Autodesk Inventor part; units mm, degrees
ref_plane "YZ Plane" through (0, 0, 0) normal (1, 0, 0) x (0, 1, 0)
ref_plane "XZ Plane" through (0, 0, 0) normal (0, 1, 0) x (-1, 0, 0)
ref_plane "XY Plane" through (0, 0, 0) normal (0, 0, 1) x (1, 0, 0)
sketch "Sketch1" plane through (0, 0, 0) normal (0, 1, 0) x (-1, 0, 0)
  line L0 (0.3746, 1.6788) -> (0.3747, -4.4196)
  line L1 (3.5497, -7.5946) -> (5.0483, -7.5946)
  arc A0 (7.6772, -6.364) -> (5.0483, -6.4323) centre (6.3183, -4.6863) ccw
  line L2 (7.6772, -7.5946) -> (20.7963, -7.5946)
  arc A1 (23.4251, -6.4323) -> (20.7962, -6.364) centre (22.1552, -4.6863) ccw
  line L3 (23.4252, -7.5946) -> (24.9238, -7.5946)
  line L4 (20.7963, 66.2432) -> (7.6772, 66.2432)
  arc A2 (5.0483, 65.0809) -> (7.6772, 65.0126) centre (6.3183, 63.3349) ccw
  line L5 (5.0483, 66.2432) -> (3.5496, 66.2432)
  line L6 (24.9237, 66.2432) -> (23.4252, 66.2432)
  arc A3 (20.7962, 65.0126) -> (23.4251, 65.0809) centre (22.1552, 63.3349) ccw
  circle A4 centre (14.2367, 45.0719) radius 6.9278
  arc A5 (1.9876, 15.9067) -> (5.1626, 12.7318) centre (5.1626, 15.9067) ccw
  line L7 (5.1626, 12.7318) -> (23.3109, 12.7318)
  arc A6 (23.3109, 12.7318) -> (26.4859, 15.9068) centre (23.3109, 15.9068) ccw
  line L8 (26.4859, 15.9068) -> (26.4859, 45.1707)
  arc A7 (26.4859, 45.1707) -> (1.9876, 45.1707) centre (14.2367, 45.0719) ccw
  line L9 (1.9876, 45.1707) -> (1.9876, 15.9067)
  arc A8 (27.813, 45.1759) -> (0.6604, 45.1759) centre (14.2367, 45.0719) ccw
  circle A9 centre (14.2367, 45.0719) radius 6.9278
  line L10 (0.3746, 66.2432) -> (13.2207, 66.2432)
  line L11 (13.2207, 66.2432) -> (13.2207, 60.019)
  line L12 (13.2207, 60.019) -> (0.3746, 60.019)
  line L13 (0.3746, 60.019) -> (0.3746, 66.2432)
  line L14 (0.3746, 60.019) -> (13.2207, 60.019)
  line L15 (13.2207, 60.019) -> (13.2207, 59.1663)
  line L16 (13.2207, 59.1663) -> (0.3746, 59.1663)
  line L17 (0.3746, 59.1663) -> (0.3746, 60.019)
  line L18 (14.2367, 45.0719) -> (14.2367, 66.2432)
  line L19 (28.0988, 66.2432) -> (15.2527, 66.2432)
  line L20 (15.2527, 66.2432) -> (15.2527, 60.019)
  line L21 (28.0988, 60.019) -> (28.0988, 66.2432)
  line L22 (28.0988, 60.019) -> (15.2527, 60.019)
  line L23 (15.2527, 60.019) -> (15.2527, 59.1663)
  line L24 (15.2527, 59.1663) -> (28.0988, 59.1663)
  line L25 (28.0988, 59.1663) -> (28.0988, 60.019)
  circle A10 centre (6.3183, 63.3349) radius 2.159
  circle A11 centre (22.1552, 63.3349) radius 2.159
  line L26 (0.3746, 66.2432) -> (0.3746, -7.5946)
  line L27 (0.3746, 29.3243) -> (28.0988, 29.3243)
  line L28 (20.7963, -7.5946) -> (7.6772, -7.5946)
  arc A12 (7.6772, -6.364) -> (5.0483, -6.4323) centre (6.3182, -4.6863) ccw
  line L29 (5.0483, -7.5946) -> (3.5497, -7.5946)
  line L30 (24.9238, -7.5946) -> (23.4252, -7.5946)
  arc A13 (23.4251, -6.4323) -> (20.7962, -6.364) centre (22.1551, -4.6863) ccw
  line L31 (0.3746, -7.5946) -> (13.2207, -7.5946)
  line L32 (13.2207, -7.5946) -> (13.2207, -1.3704)
  line L33 (13.2207, -1.3704) -> (0.3746, -1.3704)
  line L34 (0.3746, -1.3704) -> (0.3746, -7.5946)
  line L35 (0.3746, -1.3704) -> (13.2207, -1.3704)
  line L36 (13.2207, -1.3704) -> (13.2207, -0.5177)
  line L37 (13.2207, -0.5177) -> (0.3746, -0.5177)
  line L38 (0.3746, -0.5177) -> (0.3746, -1.3704)
  line L39 (28.0988, -1.3704) -> (28.0988, -7.5946)
  line L40 (28.0988, -7.5946) -> (15.2527, -7.5946)
  line L41 (15.2527, -7.5946) -> (15.2527, -1.3704)
  line L42 (28.0988, -1.3704) -> (15.2527, -1.3704)
  line L43 (15.2527, -0.5177) -> (28.0988, -0.5177)
  line L44 (15.2527, -1.3704) -> (15.2527, -0.5177)
  line L45 (28.0988, -0.5177) -> (28.0988, -1.3704)
  circle A14 centre (6.3182, -4.6863) radius 2.159
  circle A15 centre (22.1551, -4.6863) radius 2.159
  line L46 (28.0988, -7.5946) -> (15.2527, -7.5946)
  line L47 (15.2527, -7.5946) -> (15.2527, -1.3704)
  line L48 (15.2527, -1.3704) -> (28.0988, -1.3704)
  line L49 (28.0988, -1.3704) -> (28.0988, -7.5946)
  line L50 (13.2207, -7.5946) -> (0.3746, -7.5946)
  line L51 (0.3746, -7.5946) -> (0.3746, -1.3704)
  line L52 (0.3746, -1.3704) -> (13.2207, -1.3704)
  line L53 (13.2207, -1.3704) -> (13.2207, -7.5946)
  line L54 (28.0988, 66.2432) -> (15.2527, 66.2432)
  line L55 (15.2527, 66.2432) -> (15.2527, 60.019)
  line L56 (15.2527, 60.019) -> (28.0988, 60.019)
  line L57 (28.0988, 60.019) -> (28.0988, 66.2432)
  point P0 (0, 0)
  point P1 (0, 20.6785)
  point P2 (14.2367, -7.5946)
extrude "Extrusion1" add sketch "Sketch1" along normal blind 1 contours L41 L42 L39 L40 L3 L2 | L4 L19 L6 L21 L22 L20 | L33 L32 L2 L31 L1 L26 L0 | L13 L10 L5 L4 L11 L12
sketch "Sketch2" plane through (0, 0, 0) normal (0, -1, 0) x (1, 0, 0)
  circle A0 centre (-22.1552, 63.3349) radius 2.159
  line L0 (-28.0988, 66.2432) -> (-15.2527, 66.2432)
  line L1 (-28.0988, 60.019) -> (-28.0988, 66.2432)
  line L2 (-15.2527, 60.019) -> (-28.0988, 60.019)
  line L3 (-15.2527, 66.2432) -> (-15.2527, 60.019)
  circle A1 centre (-6.3183, 63.3349) radius 2.159
  line L4 (-0.3746, 66.2432) -> (-0.3746, 60.019)
  line L5 (-13.2207, 66.2432) -> (-0.3746, 66.2432)
  line L6 (-13.2207, 60.019) -> (-13.2207, 66.2432)
  line L7 (-0.3746, 60.019) -> (-13.2207, 60.019)
  circle A2 centre (-22.1551, -4.6863) radius 2.159
  line L8 (-15.2527, -1.3704) -> (-15.2527, -7.5946)
  line L9 (-28.0988, -1.3704) -> (-15.2527, -1.3704)
  line L10 (-28.0988, -7.5946) -> (-28.0988, -1.3704)
  line L11 (-15.2527, -7.5946) -> (-28.0988, -7.5946)
  line L12 (-28.0988, 60.019) -> (-0.3746, 60.019)
  line L13 (-0.3746, 60.019) -> (-0.3746, 59.13)
  line L14 (-0.3746, 59.13) -> (-28.0988, 59.13)
  line L15 (-28.0988, 59.13) -> (-28.0988, 60.019)
  line L16 (-28.0988, -1.3704) -> (-0.3746, -1.3704)
  line L17 (-0.3746, -1.3704) -> (-0.3746, -0.4814)
  line L18 (-0.3746, -0.4814) -> (-28.0988, -0.4814)
  line L19 (-28.0988, -0.4814) -> (-28.0988, -1.3704)
  point P0 (0, 0)
  dimension "d2" = 0.889
  dimension "d3" = 0.889
extrude "Extrusion2" add sketch "Sketch2" against normal blind 8.8392 contours L2 L12 L7 L13 L14 L15 | L9 L19 L18 L17 L16
sketch "Sketch3" plane through (0, 8.8392, 0) normal (0, 1, 0) x (1, 0, 0)
  line L0 (-0.3746, 1.3704) -> (-28.0988, 1.3704)
  line L1 (-28.0988, 1.3704) -> (-28.0988, -60.019)
  line L2 (-28.0988, -60.019) -> (-0.3746, -60.019)
  line L3 (-0.3746, -60.019) -> (-0.3746, 1.3704)
  point P0 (0, 0)
extrude "Extrusion3" add sketch "Sketch3" along normal blind 1
fillet "Fillet1" radius 2.032 8 edges at (-28.0988, 0.5, 66.2432) (-15.2527, 0.5, 66.2432) (-13.2207, 0.5, 66.2432) (-0.3746, 0.5, 66.2432) (-0.3746, 0.5, -7.5946) (-13.2207, 0.5, -7.5946) (-15.2527, 0.5, -7.5946) (-28.0988, 0.5, -7.5946)
fillet "Fillet2" radius 1.016 4 edges at (-13.2207, 0.5, -1.3704) (-15.2527, 0.5, -1.3704) (-15.2527, 0.5, 60.019) (-13.2207, 0.5, 60.019)
extrude "Extrusion4" cut sketch "Sketch1" along normal blind 127 contours A4
sketch "Sketch4" plane through (0, 9.8392, 0) normal (0, 1, 0) x (1, 0, 0)
  circle A0 centre (-14.2367, -45.0719) radius 6.9278
  line L0 (-28.0988, 1.3704) -> (-28.0988, -60.019)
  circle A1 centre (-14.2367, -45.0719) radius 4.0005
  circle A2 centre (-14.2367, -13.0679) radius 4.0005
  line L1 (-14.2367, -13.0679) -> (-14.2367, -5.0669)
  circle A3 centre (-14.2367, -5.0669) radius 1.8542
  circle A4 centre (-22.2377, -13.0679) radius 1.8542
  circle A5 centre (-14.2367, -21.0689) radius 1.8542
  circle A6 centre (-6.2357, -13.0679) radius 1.8542
  point P0 (0, 0)
  dimension "d12" = 8.001
  dimension "d15" = 32.004
  dimension "d20" = 8.001
  dimension "d21" = 3.7084
  dimension "d24" = 360
extrude "Extrusion5" cut sketch "Sketch4" against normal blind 127 contours A3 | A4 | A5 | A6
properties part number "Quarter-Scale Servo Front Mount Bracket"
For this review, take the finished solid that the model builds, in its own axes (mm). A direction names the side the tool comes from. Give positions to 0.01 mm unless a question says otherwise; leave off trailing zeros. Loops run counter-clockwise (first coordinate to the right, second up) from the corner with the lowest first, then second, coordinate; pieces in that order, holes last. Notation, with made-up numbers: (0.25, -37) -> (34.25, -37) arc R35 ccw to (34.25, -1) -> close; hole circle Ø3 at (-22, 40). An arc over 180 degrees is marked (long way). One line per question, with ' | ' between items.
1) To check wall thickness, follow probe 1 along Z at (x, y) = (-3.75, 5.25); probe 2 along Y at (x, z) = (-24.75, 0.5); probe 3 along Y at (x, z) = (-19, -2.5). State the ranges of each line that lie inside material, in increasing order.
Resolved:
probe 1: z = -1.37 to -0.48, 59.13 to 60.02 | probe 2: y = 8.84 to 9.84 | probe 3: y = 0 to 1
2) For faces 4 (the flat face through (-7, 1, 61)), 5 (the flat face through (-14, 4, 59.13)), 6 (the flat face through (-14, 6, -1.37)), 7 (the cylindrical face through (-15.9, 0.5, 65.7)), list the 3-axis set-ups (+Z, -Z, +X, -X, +Y, -Y) from which the entire face can be reached by the end or side of a thin tool; tool diameter is ignored.
Resolved:
face 4: +Z, +X, -X, +Y | face 5: +X, -X, -Y | face 6: -Z, +X, -X, +Y | face 7: +Z, +Y, -Y
3) Insertion check: pin 1 Ø2.5 at (x, z) = (-22.16, -4.69) entering from +Y; pin 2 Ø1.5 at (x, z) = (-15.5, 34) entering from -Y; pin 3 Ø3 at (x, y) = (-12, 4.5) entering from -Z; pin 4 Ø1.9 at (x, z) = (-9, -4.5) entering from +Y. Each pin has a flat end and moves straight along its axis. Give the tip position at first contact, or say it passes through.
Resolved:
pin 1: passes through | pin 2: stops at y = 8.84 | pin 3: stops at z = -1.37 | pin 4: stops at y = 1
4) We need section D-D (z = 31). Write out the cut boundary in (x, y), plus the area to 3 significant figures.
Resolved:
outline: (-28.1, 8.84) -> (-0.37, 8.84) -> (-0.37, 9.84) -> (-28.1, 9.84) -> close | area: 27.7 mm2
5) The part is to be moulded in two halves that separate along Z. For faces 1 (the cylindrical face through (-27.52, 0.51, 65.63)), 2 (the cylindrical face through (-17.43, 9.33, 51.22)), 3 (the flat face through (-14, 0, -1)), say which applies: +Z half, -Z half, draft (parallel to the pull), parting line (faces both ways), or undercut.
Resolved:
face 1: +Z half | face 2: undercut | face 3: draft
6) We need section B-B (z = 39.5). Write out the cut boundary in (x, y).
Resolved:
outline: (-28.1, 8.84) -> (-18.35, 8.84) -> (-18.35, 9.84) -> (-28.1, 9.84) -> close; (-10.12, 8.84) -> (-0.37, 8.84) -> (-0.37, 9.84) -> (-10.12, 9.84) -> close
7) We need section C-C (x = -6). Write out the cut boundary in (y, z), plus the area to 3 significant figures.
Resolved:
outline: (0, -7.59) -> (1, -7.59) -> (1, -6.82) -> (0, -6.82) -> close; (0, -2.55) -> (1, -2.55) -> (1, -1.37) -> (9.84, -1.37) -> (9.84, 11.23) -> (8.84, 11.23) -> (8.84, -0.48) -> (0, -0.48) -> close; (0, 59.13) -> (8.84, 59.13) -> (8.84, 14.91) -> (9.84, 14.91) -> (9.84, 60.02) -> (1, 60.02) -> (1, 61.2) -> (0, 61.2) -> close; (0, 65.47) -> (1, 65.47) -> (1, 66.24) -> (0, 66.24) -> close | area: 77.3 mm2
8) We need section A-A (y = 2.5). Write out the cut boundary in (x, z).
Resolved:
outline: (-28.1, -1.37) -> (-0.37, -1.37) -> (-0.37, -0.48) -> (-28.1, -0.48) -> close; (-28.1, 59.13) -> (-0.37, 59.13) -> (-0.37, 60.02) -> (-28.1, 60.02) -> close
